```python
from build123d import *

# Parameters (mm, degrees)
F1_DEPTH = 25.4
F2_DEPTH = 25.4
F3_DEPTH = 25.4


with BuildPart() as f1:
    # F0 (on Right) → F1 (new body, symmetric)
    with BuildSketch(Plane.YZ):
        Polygon((47.677338, 12.679111), (46.949221, 0), (61.328525, 6.781631), (60.887855, 19.032789), align=None)
    extrude(amount=F1_DEPTH, both=True)

    # F0 (on Right) → F2 (join, symmetric)
    with BuildSketch(Plane.YZ):
        Polygon((29.342864, 50.8), (28.977855, 38.105246), (46.949221, 0), (47.677338, 12.679111), align=None)
    extrude(amount=F2_DEPTH, both=True)

    # F0 (on Right) → F3 (join, symmetric)
    with BuildSketch(Plane.YZ):
        Polygon((-12.7, 0), (0, 0), (28.977855, 38.105246), (29.342864, 50.8), align=None)
    extrude(amount=F3_DEPTH, both=True)


solid = f1.part
```
Input: part model. Units: mm. Frame: model coordinates. A direction names the side the tool comes from. Give positions to 0.01 mm unless a question says otherwise; leave off trailing zeros. Write each loop counter-clockwise with the first axis right and the second up, starting at its lowest first coordinate (ties: lowest second). Pieces come first, ordered by that corner, then holes. Notation, with made-up numbers: (25.25, -39.5) - (52.25, -39.5) arc R29 ccw to (52.25, -1.5) - close; hole circle Ø3 at (20, 16.25). An arc over 180 degrees is marked (long way). Write item = value, one per line. Start each with the question number.
1. Ray query, L1, parallel to Y at x = 22.5, z = 17.5; L2, parallel to Y at x = 2.5, z = 33; L3, parallel to Y at x = -20.5, z = 35. Return the intervals inside material, ascending.
2. Section query C-C, the plane z = 29. Output: boundary loops of the cut face in (x, y).
3. Section query B-B, the plane z = 16. Output: boundary loops of the cut face in (x, y), then the cut area to 3 significant figures.
4. Access query for faces 4 (the flat face through (0, -6, 0)), 5 (the flat face through (0.36, 14.29, 18.79)), 6 (the flat face through (0.36, 38.64, 31.47)). Directions: +Z, -Z, +X, -X, +Y, -Y. A direction counts if a zero-diameter tool reaches every point of the face in a straight line with its end or side. Return the directions, or none.
5. Section query A-A, the plane x = -16. Output: boundary loops of the cut face in (y, z), then the cut area to 3 significant figures.
6. Section query D-D, the plane y = 27.5. Output: boundary loops of the cut face in (x, z), then the cut area to 4 significant figures.
7. First-contact query: pin 1 Ø12 at (x, y) = (20, 52) entering from +Z; pin 2 Ø2 at (x, y) = (-12, 8.5) entering from -Z; pin 3 Ø10 at (x, z) = (8, 17) entering from +Y. Flat tips, straight axial feed; report the tip coordinate or a pass-through.
8. Mould query, pull axis Y, two halves, no side actions, for faces 1 (the flat face through (25.4, 19, 26)), 2 (the flat face through (0.356, 54.038, 3.343)), 3 (the flat face through (0.356, 37.838, 19.319)). Classes: released by +Y, released by -Y, zero draft, split by the parting line, or undercut.
Check sheet entries:
q1.L1 = 1.78 to 13.31, 38.7 to 45.36, 57.7 to 60.94
q1.L2 = 14.61 to 25.1, 31.39 to 37.9
q1.L3 = 16.27 to 26.62, 30.44 to 36.94
q2.outline = (-25.4, 11.3) - (25.4, 11.3) - (25.4, 22.05) - (-25.4, 22.05) - close; (-25.4, 33.27) - (25.4, 33.27) - (25.4, 39.83) - (-25.4, 39.83) - close
q3.outline = (-25.4, 0.54) - (25.4, 0.54) - (25.4, 12.17) - (-25.4, 12.17) - close; (-25.4, 39.4) - (25.4, 39.4) - (25.4, 46.08) - (-25.4, 46.08) - close; (-25.4, 54.58) - (25.4, 54.58) - (25.4, 61) - (-25.4, 61) - close
q3.area = 1,260 mm2
q4.face_4 = -Z, +X, -X, +Y, -Y
q4.face_5 = -Z, +X, -X
q4.face_6 = +Z, +X, -X
q5.outline = (-12.7, 0) - (0, 0) - (28.98, 38.11) - (46.95, 0) - (61.33, 6.78) - (60.89, 19.03) - (47.68, 12.68) - (29.34, 50.8) - close
q5.area = 922 mm2
q6.outline = (-25.4, 36.16) - (25.4, 36.16) - (25.4, 48.57) - (-25.4, 48.57) - close
q6.area = 630.5 mm2
q7.pin_1 = 17.64
q7.pin_2 = 9.86
q7.pin_3 = 61.14
q8.face_1 = zero draft
q8.face_2 = released by +Y
q8.face_3 = undercut
